```python
from build123d import *

# Parameters (mm, degrees)
BOSS_EXTRUDE1_DEPTH  = 25
SKETCH3_R            = 2.8
BOSS_EXTRUDE2_DEPTH  = 69
CUT_EXTRUDE2_DEPTH   = 23
SKETCH9_R            = 2.311028434
BOSS_EXTRUDE3_DEPTH  = 20
FILLET1_R            = 8
SKETCH10_R           = 0.75
CUT_EXTRUDE4_DEPTH   = 2
LPATTERN2_COUNT      = 2
LPATTERN2_PITCH      = 2
LPATTERN2_COUNT_DIR2 = 4
LPATTERN2_PITCH_DIR2 = 18.5
SKETCH11_R           = 0.75
CUT_EXTRUDE5_DEPTH   = 2
SKETCH13_W           = 4
SKETCH13_H           = 1
BOSS_EXTRUDE4_DEPTH  = 3
SKETCH14_R           = 1.078343224
CUT_EXTRUDE6_DEPTH   = 2
LPATTERN3_COUNT      = 2
LPATTERN3_PITCH      = 60
LPATTERN3_COUNT_DIR2 = 2
LPATTERN3_PITCH_DIR2 = 82
LPATTERN4_COUNT      = 2
LPATTERN4_PITCH      = 60
LPATTERN4_COUNT_DIR2 = 2
LPATTERN4_PITCH_DIR2 = 82


with BuildPart() as part:
    # Sketch2 → Boss-Extrude1 (new body)
    with BuildSketch(Plane(origin=(0, 0, 0), x_dir=(1, 0, 0), z_dir=(0, 1, 0))):
        Polygon((0, 0), (79, 0), (79, 85), (74, 85), (74, 70), (60.5, 70), (60.5, 85), (55.5, 85), (55.5, 70), (42, 70), (42, 85), (37, 85), (37, 70), (23.5, 70), (23.5, 85), (18.5, 85), (18.5, 70), (5, 70), (5, 85), (0, 85), (0, 50), (15, 50), (15, 30), (0, 30), align=None)
    extrude(amount=BOSS_EXTRUDE1_DEPTH)

    # Sketch3 → Boss-Extrude2 (add)
    with BuildSketch(Plane.ZY.offset(-74)):
        with Locations((-79, 12.5)):
            Circle(SKETCH3_R)
    extrude(amount=BOSS_EXTRUDE2_DEPTH)

    # Sketch4 → Cut-Extrude2 (cut)
    with BuildSketch(Plane(origin=(0, 25, 0), x_dir=(1, 0, 0), z_dir=(0, 1, 0))):
        Polygon((1.5, 68.5), (1.5, 51.5), (16.5, 51.5), (16.5, 28.5), (1.5, 28.5), (1.5, 1.5), (77.5, 1.5), (77.5, 68.5), align=None)
    extrude(amount=-CUT_EXTRUDE2_DEPTH, mode=Mode.SUBTRACT)

    # Sketch9 → Boss-Extrude3 (add)
    with BuildSketch(Plane.XY.offset(-50)):
        with Locations((7.5, 12.5)):
            Circle(SKETCH9_R)
    extrude(amount=BOSS_EXTRUDE3_DEPTH)

    # Fillet1
    fillet1_edges = [part.edges().sort_by_distance(p)[0] for p in [
        (76.5, 25, -85),
        (2.5, 0, -85),
        (21, 0, -85),
        (39.5, 0, -85),
        (58, 0, -85),
        (76.5, 0, -85),
        (58, 25, -85),
        (39.5, 25, -85),
        (21, 25, -85),
        (2.5, 25, -85),
    ]]
    fillet(fillet1_edges, radius=FILLET1_R)

    # Sketch10 → Cut-Extrude4 (cut)
    with BuildSketch(Plane.XY.offset(-68.5)):
        with Locations((11.25, 8)):
            Circle(SKETCH10_R)
    cut_extrude4 = extrude(amount=-CUT_EXTRUDE4_DEPTH, mode=Mode.SUBTRACT)

    # LPattern2: Cut-Extrude4 2 × 4
    with Locations(*[(j * LPATTERN2_PITCH_DIR2, 0, i * LPATTERN2_PITCH) for i in range(LPATTERN2_COUNT) for j in range(LPATTERN2_COUNT_DIR2) if (i, j) != (0, 0)]):
        add(cut_extrude4, mode=Mode.SUBTRACT)

    # Sketch11 → Cut-Extrude5 (cut)
    with BuildSketch(Plane(origin=(16.5, 0, 0), x_dir=(0, 0, -1), z_dir=(1, 0, 0))):
        with Locations((40, 9)):
            Circle(SKETCH11_R)
    extrude(amount=-CUT_EXTRUDE5_DEPTH, mode=Mode.SUBTRACT)

    # Sketch13 → Boss-Extrude4 (add)
    with BuildSketch(Plane(origin=(79, 0, 0), x_dir=(0, 0, -1), z_dir=(1, 0, 0))):
        with Locations((5, 24.5)):
            Rectangle(SKETCH13_W, SKETCH13_H)
    boss_extrude4 = extrude(amount=BOSS_EXTRUDE4_DEPTH)

    # Sketch14 → Cut-Extrude6 (cut, through all)
    with BuildSketch(Plane(origin=(0, 24, 0), x_dir=(-1, 0, 0), z_dir=(0, -1, 0))):
        with Locations((-80.5, 5)):
            Circle(SKETCH14_R)
    cut_extrude6 = extrude(amount=-CUT_EXTRUDE6_DEPTH, mode=Mode.SUBTRACT)

    # LPattern3: Boss-Extrude4 2 × 2
    with Locations(*[(-j * LPATTERN3_PITCH_DIR2, 0, -i * LPATTERN3_PITCH) for i in range(LPATTERN3_COUNT) for j in range(LPATTERN3_COUNT_DIR2) if (i, j) != (0, 0)]):
        add(boss_extrude4)

    # LPattern4: Cut-Extrude6 2 × 2
    with Locations(*[(-j * LPATTERN4_PITCH_DIR2, 0, -i * LPATTERN4_PITCH) for i in range(LPATTERN4_COUNT) for j in range(LPATTERN4_COUNT_DIR2) if (i, j) != (0, 0)]):
        add(cut_extrude6, mode=Mode.SUBTRACT)


solid = part.part
```
Geometry check sheet. Reference: the model listing, model coordinates, mm. A direction names the side the tool comes from. Coordinates: 2 decimals unless noted, no trailing zeros. Order: outer loops, then holes, each group sorted by start corner. A loop starts at its lowest first (then second) coordinate and runs counter-clockwise, first axis right, second up.
Item 1: Section check C-C (z = -46.5). Enter the section's corners in (x, y), plus the area to 3 significant figures.
Item 2: Tool access check on faces 1 (the flat face through (40, 14, -68.5)), 2 (the cylindrical face through (20.965, 2.281, -82.594)), 3 (the cylindrical face through (67.34, 13.34, -76.33)). Record the directions out of +Z, -Z, +X, -X, +Y, -Y that give a thin tool (end or side, any length) a straight path to the whole face; none if there is none.
Item 3: Section check D-D (x = -1.5). Enter the section's corners in (y, z), plus the area to 3 significant figures.
Item 4: Mould release check, pull along X, two halves, no side actions. Record for faces 4 (the cylindrical face through (76.465, 22.594, -82.719)), 5 (the cylindrical face through (81.577, 24.493, -5.047)): released by +X, released by -X, zero draft, split by the parting line, or undercut.
Item 5: Section check B-B (z = -65). Enter the section's corners in (x, y), plus the area to 3 significant figures.
Item 6: Section check A-A (x = 31.5). Enter the section's corners in (y, z), plus the area to 3 significant figures.
Item 7: Depth check by flat-ended pin: pin 1 (1.3 mm diameter, centred on x = -1.5, z = -5, fed in from +Y); pin 2 (2 mm diameter, centred on x = 66.75, y = 8, fed in from -Z); pin 3 (7.5 mm diameter, centred on y = 10.5, z = -78, fed in from +X); pin 4 (12 mm diameter, centred on y = 5, z = -62.5, fed in from -X). Enter the tip coordinate at first touch or a pass-through.
Item 8: Scan lines: line 1 along Z through (x, y) = (80.5, 24.6); line 2 along X through (y, z) = (24.8, -5); line 3 along X through (y, z) = (6, -79.5). Record each from-to range of solid material in increasing order.
Check sheet entries:
1. outline: circle Ø4.62 at (7.5, 12.5); (15, 0) - (79, 0) - (79, 25) - (77.5, 25) - (77.5, 2) - (16.5, 2) - (16.5, 25) - (15, 25) - close
1. area: 214 mm2
2. face 1: +Y
2. face 2: -Z, +X, -X, -Y
2. face 3: none
3. outline: (24, -67) - (25, -67) - (25, -66.08) - (24, -66.08) - close; (24, -63.92) - (25, -63.92) - (25, -63) - (24, -63) - close; (24, -7) - (25, -7) - (25, -6.08) - (24, -6.08) - close; (24, -3.92) - (25, -3.92) - (25, -3) - (24, -3) - close
3. area: 3.69 mm2
4. face 4: zero draft
4. face 5: undercut
5. outline: (-3, 24) - (-2.58, 24) - (-2.58, 25) - (-3, 25) - close; (-0.42, 24) - (0, 24) - (0, 0) - (79, 0) - (79, 24) - (79.42, 24) - (79.42, 25) - (77.5, 25) - (77.5, 2) - (1.5, 2) - (1.5, 25) - (-0.42, 25) - close; (81.58, 24) - (82, 24) - (82, 25) - (81.58, 25) - close
5. area: 229 mm2
6. outline: (0, -70) - (25, -70) - (25, -68.5) - (2, -68.5) - (2, -1.5) - (25, -1.5) - (25, 0) - (0, 0) - close; circle Ø5.6 at (12.5, -79)
6. area: 234 mm2
7. pin 1: passes through
7. pin 2: stops at z = -70
7. pin 3: stops at x = 79
7. pin 4: stops at x = 0
8. line 1: z = -67 to -66.08, -63.92 to -63, -7 to -6.08, -3.92 to -3
8. line 2: x = -3 to -2.58, -0.42 to 1.5, 77.5 to 79.42, 81.58 to 82
8. line 3: x = 0 to 5, 18.5 to 23.5, 37 to 42, 55.5 to 60.5, 74 to 79
